CAD build for the part. Positions are in the model's coordinates, mm. Round coordinates to 2 decimals unless told otherwise and drop trailing zeros. Order: outer loops, then holes, each group sorted by start corner. A loop starts at its lowest first (then second) coordinate and runs counter-clockwise, first axis right, second up. Notation, with made-up numbers: M 83.5,81.5 L 96.5,81.5 A16 cw 96.5,101.5 Z; hole C 45,-23 d9. An arc over 180 degrees is marked long. Answer as a JSON object with one key per item and string values.
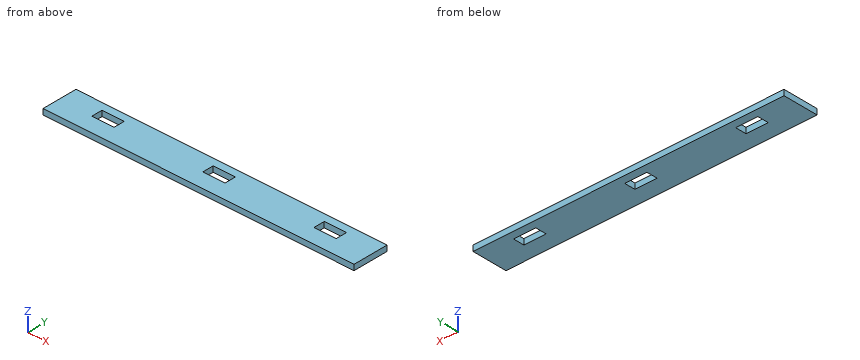
Autodesk Inventor part; units mm, degrees
ref_plane "YZ Plane" through (0, 0, 0) normal (1, 0, 0) x (0, 1, 0)
ref_plane "XZ Plane" through (0, 0, 0) normal (0, 1, 0) x (-1, 0, 0)
ref_plane "XY Plane" through (0, 0, 0) normal (0, 0, 1) x (1, 0, 0)
sketch "Sketch1" plane through (0, 0, 0) normal (0, 0, 1) x (1, 0, 0)
  line L0 (0, 0) -> (355.6, 0)
  line L1 (355.6, 0) -> (355.6, 40.64)
  line L2 (355.6, 40.64) -> (0, 40.64)
  line L3 (0, 40.64) -> (0, 0)
  line L4 (0, 31.75) -> (355.6, 31.75) construction
  line L5 (38.1, 31.75) -> (63.5, 31.75)
  line L6 (63.5, 31.75) -> (63.5, 19.05)
  line L7 (63.5, 19.05) -> (38.1, 19.05)
  line L8 (38.1, 19.05) -> (38.1, 31.75)
  line L9 (317.5, 31.75) -> (292.1, 31.75)
  line L10 (292.1, 31.75) -> (292.1, 19.05)
  line L11 (292.1, 19.05) -> (317.5, 19.05)
  line L12 (317.5, 19.05) -> (317.5, 31.75)
  line L13 (165.1, 31.75) -> (190.5, 31.75)
  line L14 (190.5, 31.75) -> (190.5, 19.05)
  line L15 (190.5, 19.05) -> (165.1, 19.05)
  line L16 (165.1, 19.05) -> (165.1, 31.75)
  dimension "d0" = 355.6
  dimension "d1" = 40.64
  dimension "d2" = 8.89
  dimension "d3" = 25.4
  dimension "d4" = 12.7
  dimension "d5" = 38.1
  dimension "d6" = 25.4
  dimension "d7" = 12.7
  dimension "d8" = 25.4
  dimension "d9" = 12.7
  dimension "d10" = 38.1
  dimension "d11" = 165.1
extrude "Extrusion1" add sketch "Sketch1" along normal blind 6.35
properties part number "latchplate" material "Aluminum 6061"
Item 1: Drop a flat-ended pin along its axis: pin 1 Ø10 at (x, y) = (153, 6.5) entering from -Z. Give the stop position or say it passes through.
Worked answers:
{"pin 1": "stops at z = 0"}
Item 2: Wall check: line 1 along X through (y, z) = (30, 2.5); line 2 along Y through (x, z) = (184.5, 4.75). Give the ranges that are in metal, low to high. Write a range as [from, to].
Worked answers:
{"line 1": "x = [0, 38.1], [63.5, 165.1], [190.5, 292.1], [317.5, 355.6]", "line 2": "y = [0, 19.05], [31.75, 40.64]"}
Item 3: Saw through at A-A on x = 179.5. List the corners of the cut face in (y, z).
Worked answers:
{"outline": "M 0,0 L 19.05,0 L 19.05,6.35 L 0,6.35 Z; M 31.75,0 L 40.64,0 L 40.64,6.35 L 31.75,6.35 Z"}
Item 4: Saw through at B-B on z = 1. List the corners of the cut face in (x, y).
Worked answers:
{"outline": "M 0,0 L 355.6,0 L 355.6,40.64 L 0,40.64 Z; hole M 38.1,19.05 L 63.5,19.05 L 63.5,31.75 L 38.1,31.75 Z; hole M 165.1,19.05 L 190.5,19.05 L 190.5,31.75 L 165.1,31.75 Z; hole M 292.1,19.05 L 317.5,19.05 L 317.5,31.75 L 292.1,31.75 Z"}
